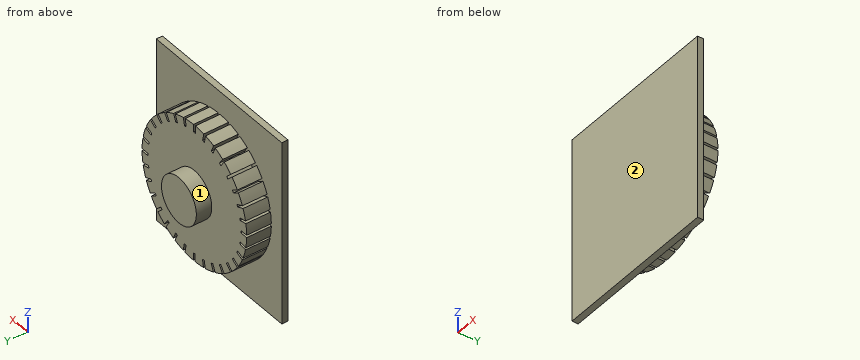
from build123d import *

# Parameters (mm, degrees)
SKETCH1_W           = 540
SKETCH1_H           = 600
BOSS_EXTRUDE1_DEPTH = 20
SKETCH2_R           = 225
BOSS_EXTRUDE2_DEPTH = 80
SKETCH3_R           = 75
BOSS_EXTRUDE3_DEPTH = 50
SKETCH4_W           = 7.808552915
SKETCH4_H           = 30.411045622
CUT_EXTRUDE2_DEPTH  = 80
CIRPATTERN1_COUNT   = 32


with BuildPart() as part:
    # Sketch1 → Boss-Extrude1 (new body)
    with BuildSketch(Plane(origin=(0, 0, 0), x_dir=(1, 0, 0), z_dir=(0, 1, 0))):
        Rectangle(SKETCH1_W, SKETCH1_H)
    extrude(amount=BOSS_EXTRUDE1_DEPTH)

    # Sketch2 → Boss-Extrude2 (add)
    with BuildSketch(Plane(origin=(0, 20, 0), x_dir=(1, 0, 0), z_dir=(0, 1, 0))):
        Circle(SKETCH2_R)
    extrude(amount=BOSS_EXTRUDE2_DEPTH)

    # Sketch3 → Boss-Extrude3 (add)
    with BuildSketch(Plane(origin=(0, 100, 0), x_dir=(1, 0, 0), z_dir=(0, 1, 0))):
        Circle(SKETCH3_R)
    extrude(amount=BOSS_EXTRUDE3_DEPTH)

    # Sketch4 → Cut-Extrude2 (cut)
    with BuildSketch(Plane(origin=(0, 100, 0), x_dir=(1, 0, 0), z_dir=(0, 1, 0))):
        with Locations((-0.422697027, -214.97303666)):
            Rectangle(SKETCH4_W, SKETCH4_H)
    cut_extrude2 = extrude(amount=-CUT_EXTRUDE2_DEPTH, mode=Mode.SUBTRACT)

    # CirPattern1: Cut-Extrude2 ×32 about axis
    cirpattern1_axis = Axis((0, 0, 0), (0, 1, 0))
    for i in range(1, CIRPATTERN1_COUNT):
        add(cut_extrude2.rotate(cirpattern1_axis, i * 360 / CIRPATTERN1_COUNT), mode=Mode.SUBTRACT)


solid = part.part
Design review of the part built by this model. Coordinates are the model's own, in mm. Face numbers are marked on the shaded views. A direction names the side the tool comes from. Give positions to 0.01 mm unless a question says otherwise; leave off trailing zeros. Loops run counter-clockwise (first coordinate to the right, second up) from the corner with the lowest first, then second, coordinate; pieces in that order, holes last. Notation, with made-up numbers: M 85.25,76 L 121.25,76 A23 ccw 121.25,114 Z; hole C 89,24 d11. An arc over 180 degrees is marked long. One line per question, with ' | ' between items. Start each with the question number.
1. Add section A-A (z = 64). Write out the cut boundary in (x, y).
2. To check wall thickness, follow L1, parallel to Z at x = 76, y = 24.5; L2, parallel to X at y = 80, z = -182.5; L3, parallel to Y at x = -125.5, z = -247. State the ranges of each line that lie inside material, in increasing order.
3. Add section C-C (x = 56). Write out the cut boundary in (y, z), plus the area to 3 significant figures.
4. Add section B-B (x = -98). Write out the cut boundary in (y, z), plus the area to 3 significant figures.
5. Insertion check: P1, Ø10, axis at y = 69, z = 177.5, coming from the +X side; P2, Ø4, axis at y = 60.5, z = 1.5, coming from the +X side; P3, Ø8.5, axis at x = 0.5, y = 66, coming from the +Z side. Each pin has a flat end and moves straight along its axis. Give the tip position at first contact, or say it passes through.
6. For the marked faces 1 and 2, list the 3-axis set-ups (+Z, -Z, +X, -X, +Y, -Y) from which the entire face can be reached by the end or side of a thin tool; tool diameter is ignored.
Worked out:
1) outline: M -270,0 L 270,0 L 270,20 L 215.71,20 L 215.71,100 L 39.1,100 L 39.1,150 L -39.1,150 L -39.1,100 L -215.71,100 L -215.71,20 L -270,20 Z
2) L1: z = -211.78 to -192.58, -184.75 to 184.75, 194.79 to 211.78 | L2: x = -131.6 to -126.13, -116.74 to 117.76, 127.15 to 131.6 | L3: y = 0 to 20
3) outline: M 0,-300 L 20,-300 L 20,-217.92 L 100,-217.92 L 100,-49.89 L 150,-49.89 L 150,49.89 L 100,49.89 L 100,217.92 L 20,217.92 L 20,300 L 0,300 Z | area: 51,900 mm²
4) outline: M 0,-300 L 20,-300 L 20,-202.54 L 100,-202.54 L 100,202.54 L 20,202.54 L 20,300 L 0,300 Z | area: 44,400 mm²
5) P1: stops at x = 144.46 | P2: stops at x = 199.77 | P3: stops at z = 224.97
6) face 1: +Y | face 2: +Z, -Z, +X, -X, -Y
